Check sheet for the modelled part. Datum: model origin and axes. Units: mm. Face numbers are marked on the shaded views. A direction names the side the tool comes from. Give positions to 0.01 mm unless a question says otherwise; leave off trailing zeros. Write each loop counter-clockwise with the first axis right and the second up, starting at its lowest first coordinate (ties: lowest second). Pieces come first, ordered by that corner, then holes. Notation, with made-up numbers: (42, -1) -> (49, -1) arc R20 cw to (49, 4) -> close; hole circle Ø6 at (68, 75.5). An arc over 180 degrees is marked (long way). Use a Markdown table: item, result. Add a question column.
1. Set-up check for the marked faces 4, 5 and 6: record each of +Z, -Z, +X, -X, +Y, -Y from which the full face is reachable in a straight line by a thin tool's end or side.
2. Scan lines: probe 1 along Z at (x, y) = (12.5, 5.5); probe 2 along X at (y, z) = (8, 8.75); probe 3 along X at (y, z) = (5.5, -0.5). Record each from-to range of solid material in increasing order. Write a range as [from, to].
3. Release check for a two-part mould opening along Z. For the marked faces 1, 2 and 3 record: released by +Z, released by -Z, zero draft, split by the parting line, or undercut.
4. Cross-section at A-A (y = 7). Enter the section's corners in (x, z) (3 decimals), then the cut area to 3 significant figures.
5. Cross-section at B-B (x = -3). Enter the section's corners in (y, z).
6. Gauge pin test, flat ends, axial feed: P1, Ø6, axis at x = 7, z = 6, coming from the +Y side; P2, Ø6, axis at x = 2, y = 7.5, coming from the +Z side; P3, Ø3, axis at x = -1.5, y = 4.5, coming from the +Z side. Record the tip position at first contact, or that the pin passes through.
7. Cross-section at D-D (z = -3.25). Enter the section's corners in (x, y).
8. Cross-section at C-C (x = 6.75). Enter the section's corners in (y, z) (3 decimals), then the cut area to 3 significant figures.
from build123d import *

# Parameters (mm, degrees)
SKETCH1_W               = 32
SKETCH1_H               = 24.5
BOSS_EXTRUDE1_DEPTH     = 10
SKETCH2_W               = 19
SKETCH2_H               = 24.5
CUT_EXTRUDE1_DEPTH      = 6
BOSS_EXTRUDE2_START     = -4
SKETCH12_W              = 32
SKETCH12_H              = 6
BOSS_EXTRUDE2_DEPTH     = 5.6
SKETCH13_W              = 9.25
SKETCH13_H              = 3.5
CUT_EXTRUDE7_DEPTH      = 25.5
SKETCH9_R               = 1.5
CUT_EXTRUDE5_DEPTH      = 8.6
CUT_EXTRUDE5_DEPTH_BACK = 5
SKETCH3_R               = 1.5
CUT_EXTRUDE2_DEPTH      = 4
SKETCH4_R               = 1.5
CUT_EXTRUDE3_DEPTH      = 7
SKETCH6_W               = 5.5
SKETCH6_H               = 12
SKETCH6_W_2             = 17
SKETCH6_H_2             = 4
CUT_EXTRUDE4_DEPTH      = 8.6
CUT_EXTRUDE4_DEPTH_BACK = 5
SKETCH16_W              = 2
SKETCH16_H              = 2
BOSS_EXTRUDE3_DEPTH     = 1.6
SKETCH17_R              = 2
CUT_EXTRUDE10_DEPTH     = 1.6
FILLET1_R               = 2
FILLET3_R               = 0.5
FILLET4_R               = 0.5
FILLET5_R               = 1
SKETCH14_R              = 1.625
CUT_EXTRUDE8_DEPTH      = 5.6


with BuildPart() as part:
    # Sketch1 → Boss-Extrude1 (new body)
    with BuildSketch(Plane(origin=(0, 0, 0), x_dir=(1, 0, 0), z_dir=(0, 1, 0))):
        Rectangle(SKETCH1_W, SKETCH1_H)
    extrude(amount=BOSS_EXTRUDE1_DEPTH)

    # Sketch2 → Cut-Extrude1 (cut)
    with BuildSketch(Plane(origin=(0, 10, 0), x_dir=(1, 0, 0), z_dir=(0, 1, 0))):
        Rectangle(SKETCH2_W, SKETCH2_H)
    extrude(amount=-CUT_EXTRUDE1_DEPTH, mode=Mode.SUBTRACT)

    # Sketch12 → Boss-Extrude2 (add)
    with BuildSketch(Plane(origin=(0, 10, 0), x_dir=(1, 0, 0), z_dir=(0, 1, 0)).offset(BOSS_EXTRUDE2_START)):
        with Locations((0, 9.25)):
            Rectangle(SKETCH12_W, SKETCH12_H)
    extrude(amount=BOSS_EXTRUDE2_DEPTH)

    # Sketch13 → Cut-Extrude7 (cut, through all)
    with BuildSketch(Plane(origin=(0, 0, -12.25), x_dir=(-1, 0, 0), z_dir=(0, 0, -1))):
        with Locations((0, 7.75)):
            Rectangle(SKETCH13_W, SKETCH13_H)
    extrude(amount=-CUT_EXTRUDE7_DEPTH, mode=Mode.SUBTRACT)

    # Sketch9 → Cut-Extrude5 (cut, two sides)
    with BuildSketch(Plane(origin=(0, 4, 0), x_dir=(1, 0, 0), z_dir=(0, 1, 0))) as cut_extrude5_sk:
        with Locations((-6.75, 8.75)):
            Circle(SKETCH9_R)
        with Locations((6.75, 8.75)):
            Circle(SKETCH9_R)
    extrude(amount=CUT_EXTRUDE5_DEPTH, mode=Mode.SUBTRACT)
    extrude(cut_extrude5_sk.sketch, amount=-CUT_EXTRUDE5_DEPTH_BACK, mode=Mode.SUBTRACT)

    # Sketch3 → Cut-Extrude2 (cut)
    with BuildSketch(Plane(origin=(0, 10, 0), x_dir=(1, 0, 0), z_dir=(0, 1, 0))):
        with Locations((-12.5, 3.25)):
            Circle(SKETCH3_R)
        with Locations((-12.5, -8.75)):
            Circle(SKETCH3_R)
        with Locations((12.5, -8.75)):
            Circle(SKETCH3_R)
        with Locations((12.5, 3.25)):
            Circle(SKETCH3_R)
        with Locations((-6.75, 8.75)):
            Circle(SKETCH3_R)
        with Locations((6.75, 8.75)):
            Circle(SKETCH3_R)
    extrude(amount=-CUT_EXTRUDE2_DEPTH, mode=Mode.SUBTRACT)

    # Sketch4 → Cut-Extrude3 (cut, through all)
    with BuildSketch(Plane(origin=(0, 6, 0), x_dir=(1, 0, 0), z_dir=(0, 1, 0))):
        with Locations((-12.5, 3.25)):
            Circle(SKETCH4_R)
        with Locations((-12.5, -8.75)):
            Circle(SKETCH4_R)
        with Locations((12.5, 3.25)):
            Circle(SKETCH4_R)
        with Locations((12.5, -8.75)):
            Circle(SKETCH4_R)
    extrude(amount=-CUT_EXTRUDE3_DEPTH, mode=Mode.SUBTRACT)

    # Sketch6 → Cut-Extrude4 (cut, two sides)
    with BuildSketch(Plane(origin=(0, 4, 0), x_dir=(1, 0, 0), z_dir=(0, 1, 0))) as cut_extrude4_sk:
        with Locations((-6.75, 0.25)):
            Rectangle(SKETCH6_W, SKETCH6_H)
        with Locations((1, -10.25)):
            Rectangle(SKETCH6_W_2, SKETCH6_H_2)
    extrude(amount=CUT_EXTRUDE4_DEPTH, mode=Mode.SUBTRACT)
    extrude(cut_extrude4_sk.sketch, amount=-CUT_EXTRUDE4_DEPTH_BACK, mode=Mode.SUBTRACT)

    # Sketch16 → Boss-Extrude3 (add)
    with BuildSketch(Plane(origin=(0, 10, 0), x_dir=(1, 0, 0), z_dir=(0, 1, 0))):
        with Locations((-15, 5.25)):
            Rectangle(SKETCH16_W, SKETCH16_H)
        with Locations((15, 5.25)):
            Rectangle(SKETCH16_W, SKETCH16_H)
    extrude(amount=BOSS_EXTRUDE3_DEPTH)

    # Sketch17 → Cut-Extrude10 (cut)
    with BuildSketch(Plane(origin=(0, 11.6, 0), x_dir=(1, 0, 0), z_dir=(0, 1, 0))):
        with Locations((-14, 4.25)):
            Circle(SKETCH17_R)
        with Locations((14, 4.25)):
            Circle(SKETCH17_R)
    extrude(amount=-CUT_EXTRUDE10_DEPTH, mode=Mode.SUBTRACT)

    # Fillet1
    fillet1_edges = [part.edges().sort_by_distance(p)[0] for p in [
        (16, 5, 12.25),
        (-16, 5, 12.25),
        (-16, 5.8, -12.25),
        (16, 5.8, -12.25),
    ]]
    fillet(fillet1_edges, radius=FILLET1_R)

    # Fillet3
    fillet3_edges = [part.edges().sort_by_distance(p)[0] for p in [
        (-9.5, 2, 5.75),
        (-9.5, 2, -6.25),
        (-4, 2, -6.25),
        (-4, 2, 5.75),
        (9.5, 2, 8.25),
        (-7.5, 2, 12.25),
        (-7.5, 2, 8.25),
        (9.5, 5, 12.25),
        (-9.5, 7, 12.25),
    ]]
    fillet(fillet3_edges, radius=FILLET3_R)

    # Fillet4
    fillet4_edges = [part.edges().sort_by_distance(p)[0] for p in [
        (-16, 11.6, -7.25),
        (0, 11.6, -12.25),
        (15.414213562, 11.6, -11.664213562),
        (-15.414213562, 11.6, -11.664213562),
        (16, 11.6, -7.25),
    ]]
    fillet(fillet4_edges, radius=FILLET4_R)

    # Fillet5
    fillet5_edges = [part.edges().sort_by_distance(p)[0] for p in [
        (-4.625, 9.5, -9.25),
        (4.625, 9.5, -9.25),
    ]]
    fillet(fillet5_edges, radius=FILLET5_R)

    # Sketch14 → Cut-Extrude8 (cut)
    with BuildSketch(Plane(origin=(0, 11.6, 0), x_dir=(1, 0, 0), z_dir=(0, 1, 0))):
        with Locations((6.75, 8.75)):
            Circle(SKETCH14_R)
        with Locations((-6.75, 8.75)):
            Circle(SKETCH14_R)
    extrude(amount=-CUT_EXTRUDE8_DEPTH, mode=Mode.SUBTRACT)


solid = part.part
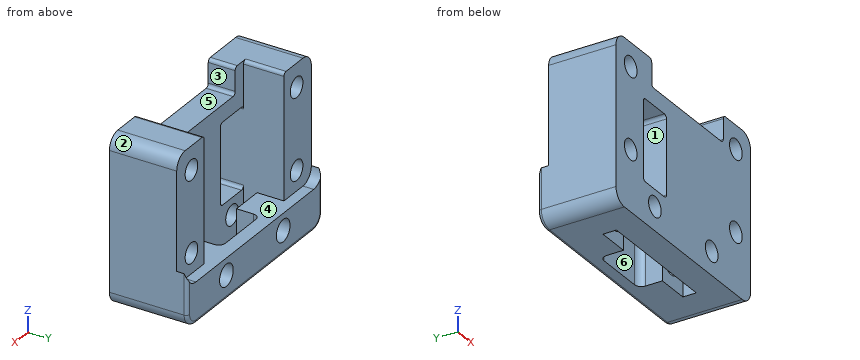
Worked answers:
| question | item | result |
|---|---|---|
| 1 | face 4 | +Z, +Y |
| 1 | face 5 | +Z, +Y, -Y |
| 1 | face 6 | +Z, -Z |
| 2 | probe 1 | z = [-12.25, -4.75], [-1.75, 7.25], [10.25, 12.25] |
| 2 | probe 2 | x = [-16, -14], [-11, -9.5], [9.5, 11], [14, 16] |
| 2 | probe 3 | x = [-16, -9.5], [9.5, 16] |
| 3 | face 1 | undercut |
| 3 | face 2 | released by +Z |
| 3 | face 3 | zero draft |
| 4 | outline | (-16, -10.25) arc R2 ccw to (-14, -12.25) -> (-4.625, -12.25) -> (-4.625, -6.25) -> (-9.5, -6.25) -> (-9.5, 11.75) arc R0.5 ccw to (-10, 12.25) -> (-14, 12.25) arc R2 ccw to (-16, 10.25) -> close; (4.625, -12.25) -> (14, -12.25) arc R2 ccw to (16, -10.25) -> (16, 10.25) arc R2 ccw to (14, 12.25) -> (10, 12.25) arc R0.5 ccw to (9.5, 11.75) -> (9.5, -6.25) -> (4.625, -6.25) -> close; hole circle Ø3 at (-12.5, -3.25); hole circle Ø3 at (-12.5, 8.75); hole circle Ø3.25 at (-6.75, -8.75); hole circle Ø3.25 at (6.75, -8.75); hole circle Ø3 at (12.5, -3.25); hole circle Ø3 at (12.5, 8.75) |
| 4 | area | 329 mm² |
| 5 | outline | (0, -12.25) -> (4, -12.25) -> (4, 8.25) -> (0, 8.25) -> close; (9.5, -12.25) -> (11.1, -12.25) arc R0.5 ccw to (11.6, -11.75) -> (11.6, -6.25) -> (9.5, -6.25) -> close |
| 6 | P1 | stops at y = 10 |
| 6 | P2 | stops at z = -6.25 |
| 6 | P3 | stops at z = 8.25 |
| 7 | outline | (-16, 0) -> (-14, 0) -> (-14, 10) -> (-16, 10) -> close; (-11, 0) -> (-9.5, 0) -> (-9.5, 10) -> (-11, 10) -> close; (-4, 0) -> (11, 0) -> (11, 10) -> (9.5, 10) -> (9.5, 4) -> (-4, 4) -> close; (14, 0) -> (16, 0) -> (16, 10) -> (14, 10) -> close |
| 8 | outline | (0, -12.25) -> (4, -12.25) -> (4, -10.25) -> (0, -10.25) -> close; (0, -7.25) -> (4, -7.25) -> (4, 8.25) -> (0, 8.25) -> close; (6, -12.25) -> (11.1, -12.25) arc R0.5 ccw to (11.6, -11.75) -> (11.6, -10.375) -> (6, -10.375) -> close; (6, -7.125) -> (11.6, -7.125) -> (11.6, -6.25) -> (6, -6.25) -> close |
| 8 | area | 85.3 mm² |
